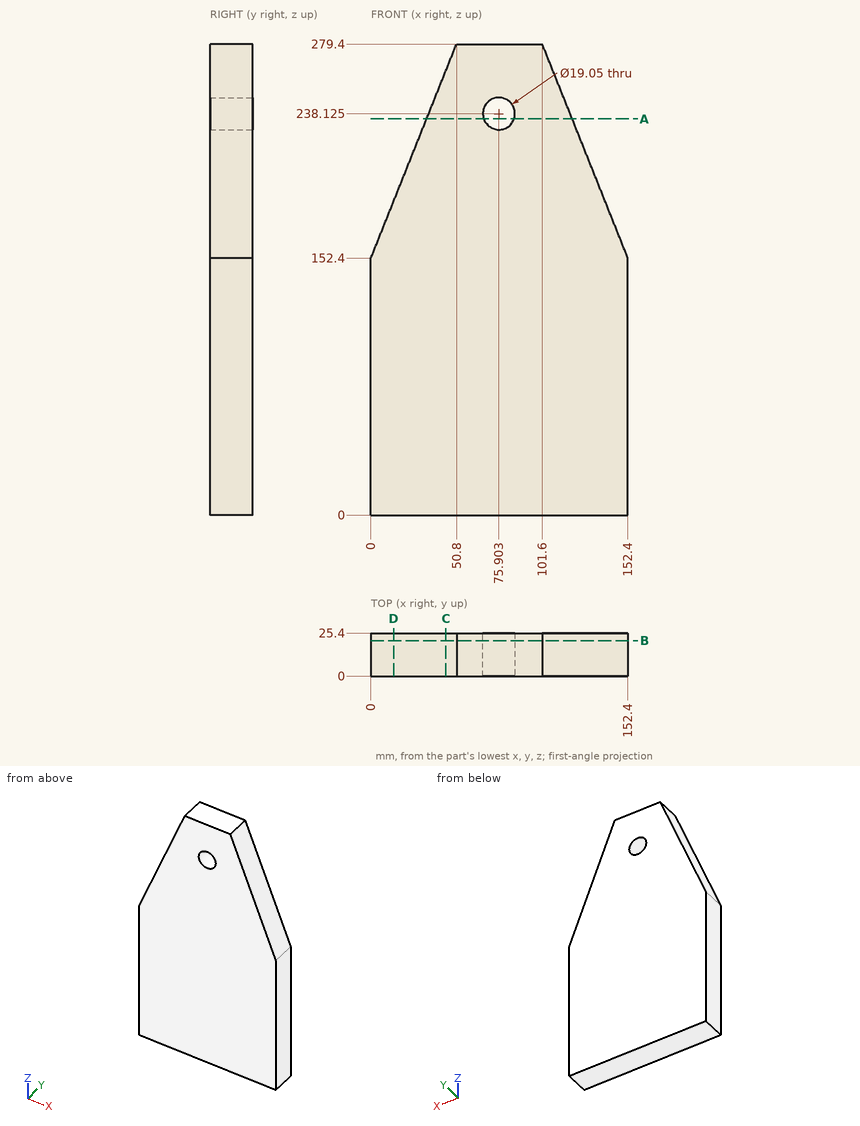
Study the drawing (mm; zero at the part's minimum x, y, z) and answer. Round coordinates to 2 decimals unless told otherwise and drop trailing zeros. Write each loop counter-clockwise with the first axis right and the second up, starting at its lowest first coordinate (ties: lowest second). Pieces come first, ordered by that corner, then holes.
1) A flat-ended cylindrical pin translates along its axis: P1, Ø15, axis at x = 75.9, z = 238.12, coming from the -Y side. Find the tip coordinate at first contact, or state that the pin passes through.
2) A cutting plane is placed at D-D on x = 13.5. Determine the outline of the cut face in (y, z).
3) Consider probe 1 along X at (y, z) = (2, 240); probe 2 along Z at (x, y) = (73, 18.25); probe 3 along X at (y, z) = (14, 184.5). Determine where each line is inside the solid, lowest interval first.
4) A cutting plane is placed at B-B on y = 21. Determine the outline of the cut face in (x, z) (3 decimals), and give its area (3 significant figures).
5) A cutting plane is placed at C-C on x = 44.5. Determine the outline of the cut face in (y, z).
6) A cutting plane is placed at A-A on z = 235. Determine the outline of the cut face in (x, y) (1 decimal), and give its area (3 significant figures).
Entries:
1. P1: passes through
2. outline: (0, 0) - (25.4, 0) - (25.4, 186.15) - (0, 186.15) - close
3. probe 1: x = 35.04 to 66.56, 85.24 to 117.36
3. probe 2: z = 0 to 229.05, 247.2 to 279.4
3. probe 3: x = 12.84 to 139.56
4. outline: (0, 0) - (152.4, 0) - (152.4, 152.4) - (101.6, 279.4) - (50.8, 279.4) - (0, 152.4) - close; hole circle Ø19.05 at (75.903, 238.125)
4. area: 35,800 mm2
5. outline: (0, 0) - (25.4, 0) - (25.4, 263.65) - (0, 263.65) - close
6. outline: (33, 0) - (66.9, 0) - (66.9, 25.4) - (33, 25.4) - close; (84.9, 0) - (119.4, 0) - (119.4, 25.4) - (84.9, 25.4) - close
6. area: 1,740 mm2
